Here's how the part is built. I have some questions about the finished solid (model axes, mm). Face numbers are marked on the shaded views. Round coordinates to 2 decimals unless told otherwise and drop trailing zeros. Loops run counter-clockwise (first coordinate to the right, second up) from the corner with the lowest first, then second, coordinate; pieces in that order, holes last. Notation, with made-up numbers: M 27,-15.75 L 31,-15.75 A22 ccw 31,5.25 Z; hole C 60,-37 d1. An arc over 180 degrees is marked long. Write each question's results on one line, items separated by ' | '. Start each with the question number.
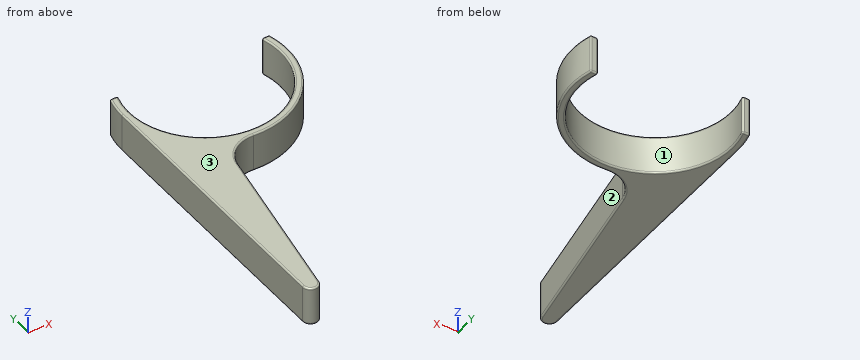
```python
from build123d import *

# Parameters (mm, degrees)
F1_DEPTH = 25
F2_R     = 1


with BuildPart() as f1:
    # F0 (on Top) → F1 (new body)
    with BuildSketch(Plane.XY):
        with BuildLine():
            Line((0, 237.1502615138), (0, 57.1502615138))
            ThreePointArc((0, 57.1502615138), (4.5642212863, 52.1692880233), (9.9240387651, 56.2820206255))
            Line((9.9240387651, 56.2820206255), (29.4444190586, 166.987598496))
            ThreePointArc((29.4444190586, 166.987598496), (36.7733002708, 179.2324763201), (50.3986553344, 183.4750265133))
            ThreePointArc((50.3986553344, 183.4750265133), (95.7512352541, 203.5193518716), (105.4293606826, 252.1502615138))
            Line((105.4293606826, 252.1502615138), (100.4293606826, 252.1502615138))
            ThreePointArc((100.4293606826, 252.1502615138), (53.7817455238, 188.1502615138), (7.134130365, 252.1502615138))
            Line((7.134130365, 252.1502615138), (2.134130365, 252.1502615138))
            ThreePointArc((2.134130365, 252.1502615138), (0.536205584, 244.7257897531), (0, 237.1502615138))
        make_face()
    extrude(amount=F1_DEPTH)

    # F2
    f2_edges = [f1.edges().sort_by_distance(p)[0] for p in [
        (19.684229, 111.63481, 25),
        (102.929361, 252.150262, 25),
        (53.781746, 188.150262, 25),
        (4.63413, 252.150262, 25),
        (0.536206, 244.72579, 25),
        (19.684229, 111.63481, 0),
        (36.7733, 179.232476, 0),
        (95.751235, 203.519352, 0),
        (36.7733, 179.232476, 25),
        (95.751235, 203.519352, 25),
        (102.929361, 252.150262, 0),
        (53.781746, 188.150262, 0),
        (0, 147.150262, 0),
        (4.63413, 252.150262, 0),
        (0.536206, 244.72579, 0),
        (4.564221, 52.169288, 0),
        (105.429361, 252.150262, 12.5),
        (100.429361, 252.150262, 12.5),
        (7.13413, 252.150262, 12.5),
        (2.13413, 252.150262, 12.5),
        (0, 147.150262, 25),
        (4.564221, 52.169288, 25),
    ]]
    fillet(f2_edges, radius=F2_R)


solid = f1.part
```
1. For pin 1 (3 mm diameter, centred on x = 59.5, z = 18.5, fed in from -Y), with a flat end and sliding along its axis, tell me the tip position at first contact or that it passes through.
2. If we mould it in two halves opening along Y, with no side actions, what happens to the marked faces 1, 2 and 3? For each: released by +Y, released by -Y, zero draft, split by the parting line, or undercut.
3. I need wall thicknesses on line 1 along X through (y, z) = (198.5, 9.75); line 2 along X through (y, z) = (241.5, 17.75); line 3 along X through (y, z) = (90, 12). Which ranges of each line are inside material? Lowest first, please.
4. I want a section at A-A on z = 20. List the corners of the cut face in (x, y) for me.
Outcome:
1) pin 1: y = 183.53
2) face 1: undercut | face 2: released by -Y | face 3: zero draft
3) line 1: 0 to 23.66, 83.9 to 91.18 | line 2: 0.18 to 4.98, 102.59 to 107.39 | line 3: 0 to 15.87
4) outline: M 0,57.15 A5 ccw 9.92,56.28 L 29.44,166.99 A20 cw 50.4,183.48 A53.78 ccw 105.64,251.42 A1 ccw 104.67,252.15 L 101.78,252.15 A1 ccw 100.82,250.87 A49 cw long 6.74,250.87 A1 ccw 5.78,252.15 L 2.89,252.15 A1 ccw 1.93,251.42 A53.78 ccw 0,237.15 Z
